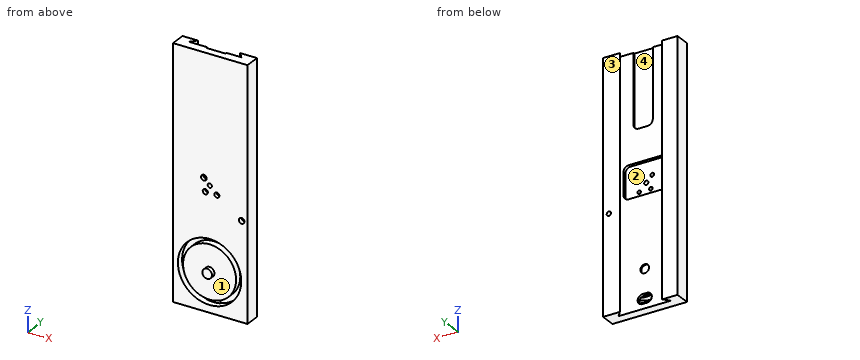
Autodesk Inventor part; units mm, degrees
ref_plane "YZ Plane" through (0, 0, 0) normal (1, 0, 0) x (0, 1, 0)
ref_plane "XZ Plane" through (0, 0, 0) normal (0, 1, 0) x (-1, 0, 0)
ref_plane "XY Plane" through (0, 0, 0) normal (0, 0, 1) x (1, 0, 0)
sketch "Sketch1" plane through (0, 0, 0) normal (0, 0, 1) x (1, 0, 0)
  line L0 (-7.7614, 0) -> (138.2386, 0)
  line L1 (138.2386, 0) -> (138.2386, 29.6)
  line L2 (-7.7614, 29.6) -> (-7.7614, 0)
  line L3 (-7.7614, 29.6) -> (22.1386, 29.6)
  line L4 (12.489, 18.1) -> (114.8883, 18.1)
  line L5 (22.1386, 29.6) -> (12.489, 18.1)
  line L6 (22.1386, 29.6) -> (41.4586, 29.6) construction
  line L7 (138.2386, 29.6) -> (105.2386, 29.6)
  line L8 (105.2386, 29.6) -> (114.8883, 18.1)
  point P0 (0, 0)
  dimension "d0" = 146
  dimension "d1" = 29.6
  dimension "d2" = 29.9
  dimension "d4" = 130
  dimension "d5" = 33
  dimension "d6" = 50
extrude "Extrusion1" add sketch "Sketch1" against normal blind 486
sketch "Sketch2" plane through (-7.7614, 29.6, 0) normal (0, 1, 0) x (1, 0, 0)
  line L0 (113, 0) -> (122.6496, 0)
  line L1 (124, 486) -> (113, 0)
  line L2 (113, 0) -> (113, 486)
  line L3 (113, 486) -> (124, 486)
  line L4 (122.6496, 0) -> (122.6496, 486)
  line L5 (113, 486) -> (113, 0)
  line L6 (146, 0) -> (146, 486)
  point P0 (7.7614, 0)
  dimension "d9" = 22
sketch "Sketch3" plane through (-7.7614, 0, 0) normal (0, -1, 0) x (1, 0, 0)
  line L0 (20.2504, -486) -> (122.6496, -486)
  line L1 (0, 0) -> (146, 0)
  circle A0 centre (71.6943, -409.4001) radius 62.1
  line L2 (71.45, -486) -> (71.4962, -471.5001)
  circle A1 centre (71.6943, -409.4001) radius 52
  circle A2 centre (71.6943, -409.4001) radius 9.51
  circle A3 centre (72.1613, -247.2004) radius 4.1
  point P0 (7.7614, 0)
  dimension "d10" = 124.2
  dimension "d11" = 14.5
  dimension "d12" = 62.1
  dimension "d13" = 104
  dimension "d14" = 19.02
  dimension "d15" = 8.2
extrude "Extrusion2" cut sketch "Sketch3" against normal blind 13 contours A0
extrude "Extrusion3" add sketch "Sketch3" along normal blind 7.5 contours A2
extrude "Extrusion4" cut sketch "Sketch3" against normal through all contours A3
sketch "Sketch4" plane through (12.489, 18.1, 0) normal (0, 1, 0) x (1, 0, 0)
  circle A0 centre (51.911, 247.2004) radius 4.1
  circle A1 centre (51.911, 247.2004) radius 9.5
  line L0 (0, 486) -> (102.3993, 486)
  line L1 (51.1996, 486) -> (51.1996, 476.6)
  arc A2 (46.6496, 476.6) -> (46.6496, 457.9) centre (46.6496, 467.25) ccw
  arc A3 (55.7496, 457.9) -> (55.7496, 476.6) centre (55.7496, 467.25) ccw
  line L2 (46.6496, 476.6) -> (55.7496, 476.6)
  line L3 (46.6496, 457.9) -> (55.7496, 457.9)
  circle A4 centre (51.1996, 411.4) radius 8.5
  point P0 (-12.489, 0)
  point P1 (51.1996, 476.6)
  dimension "d23" = 19
  dimension "d26" = 9.4
  dimension "d29" = 0
  dimension "d30" = 18.7
  dimension "d31" = 18.7
  dimension "d38" = 17
  dimension "d39" = 46.5
extrude "Extrusion5" cut sketch "Sketch4" against normal blind 3.7 contours A1
extrude "Extrusion7" cut sketch "Sketch4" against normal blind 6 contours L2 A3 L3 A2
extrude "Extrusion8" cut sketch "Sketch4" against normal blind 3 contours A4
sketch "Sketch5" plane through (-7.7614, 0, 0) normal (0, -1, 0) x (1, 0, 0)
  point P0 (7.7614, 0)
sketch "Sketch6" plane through (-7.7614, 0, 0) normal (0, -1, 0) x (1, 0, 0)
  line L0 (146, -486) -> (0, -486)
  line L1 (146, 0) -> (146, -486)
  circle A0 centre (60.5, -235.5) radius 5.5
  line L2 (0, 0) -> (0, -486)
  circle A1 centre (134.5, -295.5) radius 5.5
  point P0 (7.7614, 0)
  point P1 (86, -261)
  dimension "d45" = 11
  dimension "d46" = 60.5
  dimension "d47" = 250.5
  dimension "d48" = 11
  dimension "d49" = 190.5
  dimension "d50" = 11.5
hole "Hole1" at (126.7386, 0, -295.5) direction (0, 1, 0) diameter 8.5 end through all counterbore diameter 11 counterbore depth 8.5
hole "Hole2" at (78.2386, 0, -261) direction (0, 1, 0) diameter 7 end through all counterbore diameter 10 counterbore depth 7.5
hole "Hole3" at (52.7386, 0, -235.5) direction (0, 1, 0) diameter 7.5 end through all counterbore diameter 11 counterbore depth 7
thread "Thread1"
sketch "Sketch14" plane through (12.489, 18.1, 0) normal (0, 1, 0) x (1, 0, 0)
  circle A0 centre (51.911, 247.2004) radius 4.1 construction
  line L0 (51.911, 247.2004) -> (92.7496, 247.2004) construction
  line L1 (92.7496, 0) -> (92.7496, 486) construction
  line L2 (92.7496, 247.2004) -> (92.7496, 208.2004) construction
  line L3 (92.7496, 208.2004) -> (9.6496, 208.2004)
  line L4 (9.6496, 208.2004) -> (9.6496, 272.2004)
  line L5 (9.6496, 272.2004) -> (92.7496, 272.2004)
  line L6 (92.7496, 272.2004) -> (92.7496, 208.2004)
  point P0 (-12.489, 0)
  dimension "d82" = 39
  dimension "d83" = 83.1
  dimension "d84" = 64
extrude "Extrusion11" cut sketch "Sketch14" against normal blind 6
sketch "Sketch17" plane through (12.489, 18.1, 0) normal (0, 1, 0) x (1, 0, 0)
  line L0 (92.7496, 0) -> (92.7496, 486) construction
  line L1 (92.7496, 0) -> (73.3996, 0) construction
  line L2 (-20.2504, 0) -> (125.7496, 0) construction
  line L3 (73.3996, 0) -> (35.3996, 0)
  line L4 (35.3996, 0) -> (35.3996, 145)
  line L5 (35.3996, 145) -> (73.3996, 145)
  line L6 (73.3996, 145) -> (73.3996, 0)
  point P0 (-12.489, 0)
  dimension "d99" = 19.35
  dimension "d100" = 38
  dimension "d101" = 145
extrude "Extrusion13" cut sketch "Sketch17" against normal blind 3
sketch "Sketch18" plane through (-7.7614, 0, 0) normal (0, -1, 0) x (1, 0, 0)
  circle A0 centre (86, -261) radius 5
  point P0 (7.7614, 0)
  point P1 (63.3, -261)
  dimension "d112" = 22.7
hole "Hole5" at (55.5386, 0, -261) direction (0, 1, 0) diameter 7 end through all counterbore diameter 10 counterbore depth 7.5
fillet "Fillet1" radius 10 6 edges at (22.1386, 15.1, -208.2004) (22.1386, 15.1, -272.2004) (105.2386, 15.1, -208.2004) (105.2386, 15.1, -272.2004) (47.8886, 16.6, -145) (85.8886, 16.6, -145)
properties part number "slide ontop of saddle" material "Steel, Cast"
Build history of the part. All positions in model axes, mm. Face numbers are marked on the shaded views. A direction names the side the tool comes from. Round coordinates to 2 decimals unless told otherwise and drop trailing zeros. Write each loop counter-clockwise with the first axis right and the second up, starting at its lowest first coordinate (ties: lowest second). Pieces come first, ordered by that corner, then holes.
1) Band-saw the part on C-C, the plane z = -429.5. List the corners of the cut face in (x, y).
2) Mould opens along X. For the marked faces 1 and 2 say: +X half, -X half, draft (parallel to the pull), parting line (faces both ways), or undercut.
3) 3-axis set-ups, long thin cutter, end or side, ignore diameter. For the marked faces 3 and 4: which of +Z, -Z, +X, -X, +Y, -Y reach the whole face in a straight line?
4) Pin check, flat tips, straight feed: pin 1 (4 mm diameter, centred on x = 63, z = -460, fed in from +Y); pin 2 (3 mm diameter, centred on x = 69.5, z = -122, fed in from +Y); pin 3 (10 mm diameter, centred on x = 126.74, z = -295.5, fed in from -Y). Stop position of each tip, or through.
5) Drill centre lines: probe 1 along X at (y, z) = (11.1, -261); probe 2 along X at (y, z) = (1.5, -261); probe 3 along Z at (x, y) = (24, 8). Where is each one in solid material? Low to high.
6) Band-saw the part on A-A, the plane z = -295.5. List the corners of the cut face in (x, y).
7) Band-saw the part on B-B, the plane z = -195. List the corners of the cut face in (x, y).
Ans:
1. outline: (-7.76, 0) - (5.18, 0) - (5.18, 13) - (15.97, 13) - (15.97, 0) - (111.89, 0) - (111.89, 13) - (122.69, 13) - (122.69, 0) - (138.24, 0) - (138.24, 29.6) - (105.24, 29.6) - (114.89, 18.1) - (12.49, 18.1) - (22.14, 29.6) - (-7.76, 29.6) - close
2. face 1: draft
2. face 2: undercut
3. face 3: +Z, -Z, +X, -X, +Y
3. face 4: +Z, +Y
4. pin 1: stops at y = 12.1
4. pin 2: stops at y = 15.1
4. pin 3: stops at y = 8.5
5. probe 1: x = -7.76 to 52.04, 59.04 to 74.74, 81.74 to 138.24
5. probe 2: x = -7.76 to 50.54, 60.54 to 73.24, 83.24 to 138.24
5. probe 3: z = -486 to -456.96, -442.71 to -376.09, -361.84 to 0
6. outline: (-7.76, 0) - (121.24, 0) - (121.24, 8.5) - (122.49, 8.5) - (122.49, 29.6) - (105.24, 29.6) - (114.89, 18.1) - (12.49, 18.1) - (22.14, 29.6) - (-7.76, 29.6) - close; (130.99, 8.5) - (132.24, 8.5) - (132.24, 0) - (138.24, 0) - (138.24, 29.6) - (130.99, 29.6) - close
7. outline: (-7.76, 0) - (138.24, 0) - (138.24, 29.6) - (105.24, 29.6) - (114.89, 18.1) - (12.49, 18.1) - (22.14, 29.6) - (-7.76, 29.6) - close
